from build123d import *

# Parameters (mm, degrees)
SKETCH5_R           = 1.5875
BOSS_EXTRUDE2_DEPTH = 3.175


with BuildPart() as part:
    # Sketch5 → Boss-Extrude2 (new body)
    with BuildSketch(Plane.XY):
        with BuildLine():
            Line((-82.55, 58.42), (-82.55, 45.72))
            Line((-82.55, 45.72), (-31.848963051, 45.72))
            ThreePointArc((-31.848963051, 45.72), (-27.35883499, 43.860128061), (-25.498963051, 39.37))
            Line((-25.498963051, 39.37), (-25.498963051, 17.145))
            ThreePointArc((-25.498963051, 17.145), (-24.569027081, 14.89993597), (-22.323963051, 13.97))
            Line((-22.323963051, 13.97), (22.126036949, 13.97))
            ThreePointArc((22.126036949, 13.97), (24.37110098, 14.89993597), (25.301036949, 17.145))
            Line((25.301036949, 17.145), (25.301036949, 39.37))
            ThreePointArc((25.301036949, 39.37), (27.160908889, 43.860128061), (31.651036949, 45.72))
            Line((31.651036949, 45.72), (82.55, 45.72))
            Line((82.55, 45.72), (82.55, 58.42))
            Line((82.55, 58.42), (22.933465972, 183.638614313))
            ThreePointArc((22.933465972, 183.638614313), (0, 198.12), (-22.933465972, 183.638614313))
            Line((-22.933465972, 183.638614313), (-82.55, 58.42))
        make_face()
        with Locations((21.166666667, 18.525000034)):
            Circle(SKETCH5_R, mode=Mode.SUBTRACT)
        with Locations((-21.166666667, 18.525000034)):
            Circle(SKETCH5_R, mode=Mode.SUBTRACT)
        with Locations((-77.7875, 52.07)):
            Circle(SKETCH5_R, mode=Mode.SUBTRACT)
        with Locations((77.7875, 52.07)):
            Circle(SKETCH5_R, mode=Mode.SUBTRACT)
        with BuildLine():
            Line((-61.138040857, 73.849653578), (-27.615581335, 144.260253558))
            ThreePointArc((-27.615581335, 144.260253558), (-23.498279642, 147.671514779), (-18.235179035, 146.728833317))
            ThreePointArc((-18.235179035, 146.728833317), (-17.071685329, 145.950239821), (-15.875, 145.22369343))
            ThreePointArc((-15.875, 145.22369343), (-13.550738686, 142.899432116), (-12.7, 139.724432116))
            Line((-12.7, 139.724432116), (-12.7, 71.12))
            ThreePointArc((-12.7, 71.12), (-14.559871939, 66.629871939), (-19.05, 64.77))
            Line((-19.05, 64.77), (-55.404674364, 64.77))
            ThreePointArc((-55.404674364, 64.77), (-60.77383632, 67.729631305), (-61.138040857, 73.849653578))
        make_face(mode=Mode.SUBTRACT)
        with BuildLine():
            Line((61.138040857, 73.849653578), (27.615581335, 144.260253558))
            ThreePointArc((27.615581335, 144.260253558), (23.498279642, 147.671514779), (18.235179035, 146.728833317))
            ThreePointArc((18.235179035, 146.728833317), (17.071685329, 145.950239821), (15.875, 145.22369343))
            ThreePointArc((15.875, 145.22369343), (13.550738686, 142.899432116), (12.7, 139.724432116))
            Line((12.7, 139.724432116), (12.7, 71.12))
            ThreePointArc((12.7, 71.12), (14.559871939, 66.629871939), (19.05, 64.77))
            Line((19.05, 64.77), (55.404674364, 64.77))
            ThreePointArc((55.404674364, 64.77), (60.77383632, 67.729631305), (61.138040857, 73.849653578))
        make_face(mode=Mode.SUBTRACT)
    extrude(amount=BOSS_EXTRUDE2_DEPTH)


solid = part.part
Verification items for the finished model (mm, model axes). A direction names the side the tool comes from. Give positions to 0.01 mm unless a question says otherwise; leave off trailing zeros. Write each loop counter-clockwise with the first axis right and the second up, starting at its lowest first coordinate (ties: lowest second). Pieces come first, ordered by that corner, then holes.
(1) Cross-section at C-C (z = 0.8). State how many separate pieces and enclosed holes the cut face has, plus the area to 3 significant figures.
(2) Material ranges on line 1 (X direction, y = 71, z = 0.4); line 2 (X direction, y = 102, z = 2); line 3 (Y direction, x = 21.5, z = 1.45), recorded low to high.
(3) Gauge pin test, flat ends, axial feed: pin 1 (1.5 mm diameter, centred on x = -36, z = 1.5, fed in from +Y); pin 2 (12 mm diameter, centred on x = 47.5, y = 122.5, fed in from -Z); pin 3 (1.6 mm diameter, centred on x = 56.5, z = 1.5, fed in from -Y); pin 4 (1.5 mm diameter, centred on y = 81, z = 3, fed in from +X). Record the tip position at first contact, or that the pin passes through.
(4) Cross-section at B-B (x = -42.5). Enter the section's corners in (y, z) (3 decimals), plus the area to 3 significant figures.
(5) Cross-section at A-A (y = 98.5). Enter the section's corners in (x, z) (3 decimals).
(6) Access from +Z, -Z, +X, -X, +Y, -Y to the whole of each face (thin tool, end or side, straight path). Record for faces 5 (the face through (-52.324, 121.906, 1.565)), 6 (the face through (-14.51, 66.68, 1.57)).
(7) Mould release check, pull along X, two halves, no side actions. Record for faces 1 (the face through (-1, 87, 0)), 2 (the face through (53.16, 120.15, 1.57)), 3 (the face through (-44.611, 108.562, 1.565)), 4 (the face through (-60.725, 67.654, 1.565)): +X half, -X half, draft (parallel to the pull), parting line (faces both ways), or undercut.
Worked out:
1. separate pieces: 1
1. enclosed holes: 6
1. area: 12,000 mm2
2. line 1: x = -76.56 to -61.75, -12.7 to 12.7, 61.75 to 76.56
2. line 2: x = -61.8 to -47.74, -12.7 to 12.7, 47.74 to 61.8
2. line 3: y = 13.97 to 16.97, 20.08 to 64.77, 147.87 to 186.24
3. pin 1: stops at y = 157.77
3. pin 2: stops at z = 0
3. pin 3: stops at y = 45.72
3. pin 4: stops at x = 72.16
4. outline: (45.72, 0) - (64.77, 0) - (64.77, 3.175) - (45.72, 3.175) - close; (112.997, 0) - (142.541, 0) - (142.541, 3.175) - (112.997, 3.175) - close
4. area: 154 mm2
5. outline: (-63.468, 0) - (-49.402, 0) - (-49.402, 3.175) - (-63.468, 3.175) - close; (-12.7, 0) - (12.7, 0) - (12.7, 3.175) - (-12.7, 3.175) - close; (49.402, 0) - (63.468, 0) - (63.468, 3.175) - (49.402, 3.175) - close
6. face 5: +Z, -Z, -X, +Y
6. face 6: +Z, -Z
7. face 1: draft
7. face 2: +X half
7. face 3: undercut
7. face 4: undercut
